```python
from build123d import *

# Parameters (mm, degrees)
REVOLVE1_ANGLE     = 270
SKETCH3_R          = 5
CUT_EXTRUDE1_DEPTH = 8


with BuildPart() as part:
    # Sketch2 → Revolve1 (revolve)
    with BuildSketch(Plane(origin=(0, 0, 0), x_dir=(0, 0, -1), z_dir=(1, 0, 0))):
        Polygon((0, 0), (-8, 0), (-8, 2), (0, 4.143593539), (0, 25), (6, 25), (6, 0), (28, 0), (28, -14), (24, -14), (24, -4), (4, -4), (4, -14), (0, -14), align=None)
    revolve(axis=Axis((0, -35, 8), (0, 0, 1)), revolution_arc=REVOLVE1_ANGLE)

    # Sketch3 → Cut-Extrude1 (cut)
    with BuildSketch(Plane.XY):
        with Locations((-49.57179677, -35)):
            Circle(SKETCH3_R)
        with Locations((-35.759660433, -70.759660433)):
            Circle(SKETCH3_R)
        with Locations((-0.707106781, -86.278903551)):
            Circle(SKETCH3_R)
        with Locations((35.052553651, -72.466767214)):
            Circle(SKETCH3_R)
        with Locations((50.57179677, -37.414213562)):
            Circle(SKETCH3_R)
        with Locations((36.759660433, -1.65455313)):
            Circle(SKETCH3_R)
        with Locations((1.707106781, 13.864689989)):
            Circle(SKETCH3_R)
        with Locations((-34.052553651, 0.052553651)):
            Circle(SKETCH3_R)
    extrude(amount=-CUT_EXTRUDE1_DEPTH, mode=Mode.SUBTRACT)


solid = part.part
```
Geometry check sheet. Reference: the model listing, model coordinates, mm. A direction names the side the tool comes from. Round coordinates to 2 decimals unless told otherwise and drop trailing zeros. Order: outer loops, then holes, each group sorted by start corner. A loop starts at its lowest first (then second) coordinate and runs counter-clockwise, first axis right, second up. Notation, with made-up numbers: (40.25, 24.5) - (44.25, 24.5) arc R21 ccw to (44.25, 59.5) - close; hole circle Ø3 at (-25.75, -9). An arc over 180 degrees is marked (long way). Use a Markdown table: item, result. Add a question column.
1) Mould release check, pull along X, two halves, no side actions. Record for faces 5 (the cylindrical face through (-3.292, 13.95, -2.958)), 6 (the flat face through (-16, -50, 0)), 7 (the conical face through (-27.109, -60.377, 7.5)): released by +X, released by -X, zero draft, split by the parting line, or undercut.
2) Gauge pin test, flat ends, axial feed: P1, Ø12, axis at x = -30.5, z = 2.5, coming from the +Y side; P2, Ø11.5, axis at x = -49.57, y = -35, coming from the +Z side; P3, Ø18.5, axis at x = -14.5, y = -34, coming from the -Z side; P4, Ø5, axis at y = 20.5, z = -3.5, coming from the +X side. Record the tip position at first contact, or that the pin passes through.
3) Section check B-B (x = 42). Record the cut outline in (y, z).
4) Thickness scan on line 1 along Z through (x, y) = (-16, -8.5); line 2 along Z through (x, y) = (-22.5, 9); line 3 along X through (y, z) = (-45, -17). Record the ranges inside material, lowest first.
5) Set-up check for faces 1 (the flat face through (-28, -63, -6)), 2 (the cylindrical face through (-25.55, -58.92, 4.06)), 3 (the flat face through (0, -2, -10)), 4 (the flat face through (-14, -51, -4)): record each of +Z, -Z, +X, -X, +Y, -Y from which the full face is reachable in a straight line by a thin tool's end or side.
6) Section check A-A (z = -14.5). Record the cut outline in (x, y), then the cut area to 3 significant figures.
Established:
| question | item | result |
|---|---|---|
| 1 | face 5 | released by +X |
| 1 | face 6 | undercut |
| 1 | face 7 | split by the parting line |
| 2 | P1 | y = 19.52 |
| 2 | P2 | z = 0 |
| 2 | P3 | z = -28 |
| 2 | P4 | x = 0 |
| 3 | outline | (-77.85, -6) - (-35, -6) - (-35, 0) - (-77.85, 0) - close |
| 4 | line 1 | -28 to -24, -4 to 0 |
| 4 | line 2 | -6 to 0 |
| 4 | line 3 | -33.54 to -29.34, 29.34 to 33.54 |
| 5 | face 1 | -Z |
| 5 | face 2 | +Z |
| 5 | face 3 | +Z, -Z, +X, +Y |
| 5 | face 4 | none |
| 6 | outline | (0, -4) - (0, 0) arc R35 ccw (long way) to (35, -35) - (31, -35) arc R31 cw (long way) to start |
| 6 | area | 622 mm2 |
